Can you work these out from the model? Positions are in its coordinate system, mm. A direction names the side the tool comes from. Give positions to 0.01 mm unless a question says otherwise; leave off trailing zeros. Loops run counter-clockwise (first coordinate to the right, second up) from the corner with the lowest first, then second, coordinate; pieces in that order, holes last. Notation, with made-up numbers: (-11.75, -4.5) - (-1.75, -4.5) arc R19 ccw to (-1.75, 19.5) - close; hole circle Ø1 at (81, 60.25). An arc over 180 degrees is marked (long way). Write item = value, one per line.
from build123d import *

# Parameters (mm, degrees)
F0_R     = 31.369
F1_DEPTH = 2.54
F2_R     = 27.94
F2_R_2   = 25.4
F3_DEPTH = 15.494
F5_DEPTH = 25.4
F7_DEPTH = 20.828


with BuildPart() as f1:
    # F0 (on Top) → F1 (new body)
    with BuildSketch(Plane.XY):
        Circle(F0_R)
    extrude(amount=F1_DEPTH)

    # F2 (on Top) → F3 (join)
    with BuildSketch(Plane.XY):
        Circle(F2_R)
        Circle(F2_R_2, mode=Mode.SUBTRACT)
    extrude(amount=F3_DEPTH)

    # F4 (on face) → F5 (cut)
    with BuildSketch(Plane.XY):
        with BuildLine():
            Line((0, -0.635), (0, 0))
            Line((0, 0), (0, 0.635))
            Line((0, 0.635), (-31.330898, 0.635))
            Line((-31.330898, 0.635), (-31.362572, 0.635))
            ThreePointArc((-31.362572, 0.635), (-31.369, -0.002537), (-31.362469, -0.640074))
            Line((-31.362469, -0.640074), (-31.013001, -0.635))
            Line((-31.013001, -0.635), (0, -0.635))
        make_face()
        with BuildLine():
            Line((-31.979989, -0.649039), (-31.362469, -0.640074))
            ThreePointArc((-31.362469, -0.640074), (-31.369, -0.002537), (-31.362572, 0.635))
            Line((-31.362572, 0.635), (-31.979989, 0.635))
            Line((-31.979989, 0.635), (-31.979989, -0.649039))
        make_face()
        Polygon((0, 0.635), (0, 0), (0, -0.635), (7.969206, -0.635), (7.969206, 0.635), (4.666724, 0.635), align=None)
    extrude(amount=F5_DEPTH, mode=Mode.SUBTRACT)

    # F6 (on Top) → F7 (join)
    with BuildSketch(Plane.XY):
        with BuildLine():
            Line((18.161, -21.232562), (-18.161, -21.232562))
            ThreePointArc((-18.161, -21.232562), (0, -27.94), (18.161, -21.232562))
        make_face()
    extrude(amount=F7_DEPTH)


solid = f1.part
Q1. Which directions (+Z, -Z, +X, -X, +Y, -Y) give clear straight access to the entire face, cutting with the end or side of a thin tool? Please do faces 1 (the flat face through (10, 24, 15.494)), 2 (the flat face through (-17, -0.635, 2)), 3 (the flat face through (0, -24, 20.828)), 4 (the cylindrical face through (12.975, 21.836, 8.926)).
Output:
face_1 = +Z, +X, -X, +Y
face_2 = +Z, -Z, -X
face_3 = +Z, +X, -X, +Y, -Y
face_4 = +Z
Q2. Imagine slicing it at C-C, the plane x = 11.5. Write out the boundary of the cut face in (y, z) (3 decimals), then the cut area to 3 significant figures.
Output:
outline = (-29.185, 0) - (29.185, 0) - (29.185, 2.54) - (25.464, 2.54) - (25.464, 15.494) - (22.648, 15.494) - (22.648, 2.54) - (-21.233, 2.54) - (-21.233, 20.828) - (-25.464, 20.828) - (-25.464, 2.54) - (-29.185, 2.54) - close
area = 262 mm2
Q3. I need wall thicknesses on L1, parallel to Y at x = 0, z = 8.75; L2, parallel to Z at x = -9, y = -8; L3, parallel to Z at x = -21, y = 15. Which ranges of each line are inside material? Lowest first, please.
Output:
L1 = -27.94 to -21.23, 25.4 to 27.94
L2 = 0 to 2.54
L3 = 0 to 15.49
Q4. Imagine slicing it at D-D, the plane z = 11.5. Write out the boundary of the cut face in (x, y) (3 decimals).
Output:
outline = (-27.933, -0.635) arc R27.94 ccw (long way) to (-27.933, 0.635) - (-25.392, 0.635) arc R25.4 cw (long way) to (13.941, -21.233) - (-13.941, -21.233) arc R25.4 cw to (-25.392, -0.635) - close
Q5. Imagine slicing it at B-B, the plane y = 13.5. Write out the boundary of the cut face in (x, z).
Output:
outline = (-28.32, 0) - (28.32, 0) - (28.32, 2.54) - (24.46, 2.54) - (24.46, 15.49) - (21.52, 15.49) - (21.52, 2.54) - (-21.52, 2.54) - (-21.52, 15.49) - (-24.46, 15.49) - (-24.46, 2.54) - (-28.32, 2.54) - close
Q6. We'd pull the mould along Y, two halves only. Please class faces 5 (the flat face through (0, 2, 2.54)), 6 (the flat face through (0, -7, 0)): released by +Y, released by -Y, zero draft, split by the parting line, or undercut.
Output:
face_5 = undercut
face_6 = zero draft
Q7. For pin 1 (23.5 mm diameter, centred on x = 9.5, y = 3, fed in from +Z); pin 2 (5 mm diameter, centred on x = 12, z = 9.5, fed in from +Y); pin 3 (2 mm diameter, centred on x = 18.5, z = 2.5, fed in from +Y), each with a flat end and sliding along its axis, tell me the tip position at first contact or that it passes through.
Output:
pin_1 = 2.54
pin_2 = 26.28
pin_3 = 26.03
Q8. Imagine slicing it at A-A, the plane x = 0. Write out the boundary of the cut face in (y, z) (3 decimals).
Output:
outline = (-31.369, 0) - (-0.635, 0) - (-0.635, 2.54) - (-21.233, 2.54) - (-21.233, 20.828) - (-27.94, 20.828) - (-27.94, 2.54) - (-31.369, 2.54) - close; (0.635, 0) - (31.369, 0) - (31.369, 2.54) - (27.94, 2.54) - (27.94, 15.494) - (25.4, 15.494) - (25.4, 2.54) - (0.635, 2.54) - close
